Build history of the part. All positions in model axes, mm. A direction names the side the tool comes from. Round coordinates to 2 decimals unless told otherwise and drop trailing zeros. Write each loop counter-clockwise with the first axis right and the second up, starting at its lowest first coordinate (ties: lowest second). Pieces come first, ordered by that corner, then holes.
1) Wall check: probe 1 along Z at (x, y) = (0, -35); probe 2 along Z at (x, y) = (-6.5, -41); probe 3 along X at (y, z) = (-42, 23.5). Give the ranges that are in metal, low to high.
2) Which spindle directions (+Z, -Z, +X, -X, +Y, -Y) get a long thin tool onto all of the face, cutting with end or side? Do faces 1 (the flat face through (0, -7.5, 14)), 2 (the cylindrical face through (0.261, -39.44, 27.498)). Say none if no direction does.
3) Flat gauge pins, fed straight in: pin 1 (8 mm diameter, centred on y = -57, z = 0, fed in from +X); pin 2 (2 mm diameter, centred on x = -3, y = -25, fed in from +Z); pin 3 (5 mm diameter, centred on y = -64.5, z = 23, fed in from -X). Where does each tip first touch, or does it go through?
4) Saw through at B-B (z = 13.75). Write the cut outline in (x, y).
5) Pull direction X, two halves, no side cores. Call faces 3 (the cylindrical face through (5.19, -43.24, 3.77)), 4 (the flat face through (0, -80, 1)), 5 (the flat face through (-14.817, -39.44, 10.406)): +X half, -X half, draft (parallel to the pull), parting line (faces both ways), or undercut.
6) Saw through at A-A (x = 0). Write the cut outline in (y, z).
from build123d import *

# Parameters (mm, degrees)
F0_R     = 11.25
F1_DEPTH = 80
F2_DEPTH = 7.5
F3_R     = 5
F4_R     = 5


with BuildPart() as f1:
    # F0 (on Front) → F1 (new body)
    with BuildSketch(Plane.XZ):
        with BuildLine():
            ThreePointArc((13.75, 13.75), (9.722718, 4.027282), (0, 0))
            Line((0, 0), (17.110662, 0))
            Line((17.110662, 0), (13.427706, 16.709596))
            ThreePointArc((13.427706, 16.709596), (13.669189, 15.238546), (13.75, 13.75))
        make_face()
        Polygon((17.110662, 0), (0, 0), (-17.110662, 0), (-25, 0), (-25, -10), (25, -10), (25, 0), align=None)
        with BuildLine():
            Line((-17.110662, 0), (0, 0))
            ThreePointArc((0, 0), (-10.718137, 5.136985), (-13.427706, 16.709596))
            Line((-13.427706, 16.709596), (-17.110662, 0))
        make_face()
        with BuildLine():
            ThreePointArc((-13.427706, 16.709596), (-10.718137, 5.136985), (0, 0))
            ThreePointArc((0, 0), (9.722718, 4.027282), (13.75, 13.75))
            ThreePointArc((13.75, 13.75), (13.669189, 15.238546), (13.427706, 16.709596))
            ThreePointArc((13.427706, 16.709596), (0, 27.5), (-13.427706, 16.709596))
        make_face()
        with Locations((0, 13.75)):
            Circle(F0_R, mode=Mode.SUBTRACT)
    extrude(amount=F1_DEPTH)

    # F0 (on Front) → F2 (join)
    with BuildSketch(Plane.XZ):
        with Locations((0, 13.75)):
            Circle(F0_R)
    extrude(amount=F2_DEPTH)

    # F3
    f3_edges = [f1.edges().sort_by_distance(p)[0] for p in [
        (-17.110662, -40, 0),
        (17.110662, -40, 0),
    ]]
    fillet(f3_edges, radius=F3_R)

    # F4
    f4_edges = [f1.edges().sort_by_distance(p)[0] for p in [
        (-25, -40, 0),
        (25, -40, 0),
    ]]
    fillet(f4_edges, radius=F4_R)


solid = f1.part
Evaluation:
1. probe 1: z = -10 to 2.5, 25 to 27.5
1. probe 2: z = -10 to 4.57, 22.93 to 25.87
1. probe 3: x = -9.7 to -5.61, 5.61 to 9.7
2. face 1: -Y
2. face 2: +Z, +Y, -Y
3. pin 1: stops at x = 24.91
3. pin 2: stops at z = 27.35
3. pin 3: stops at x = -11.98
4. outline: (-14.08, -80) - (-11.25, -80) - (-11.25, -7.5) - (11.25, -7.5) - (11.25, -80) - (14.08, -80) - (14.08, 0) - (-14.08, 0) - close
5. face 3: undercut
5. face 4: draft
5. face 5: -X half
6. outline: (-80, -10) - (0, -10) - (0, 27.5) - (-80, 27.5) - (-80, 25) - (-7.5, 25) - (-7.5, 2.5) - (-80, 2.5) - close
